Source: three-view drawing plus pictorial views. Frame: mm from the lowest corner of the part. A direction names the side the tool comes from. Round coordinates to 2 decimals unless told otherwise and drop trailing zeros. Write each loop counter-clockwise with the first axis right and the second up, starting at its lowest first coordinate (ties: lowest second). Pieces come first, ordered by that corner, then holes.
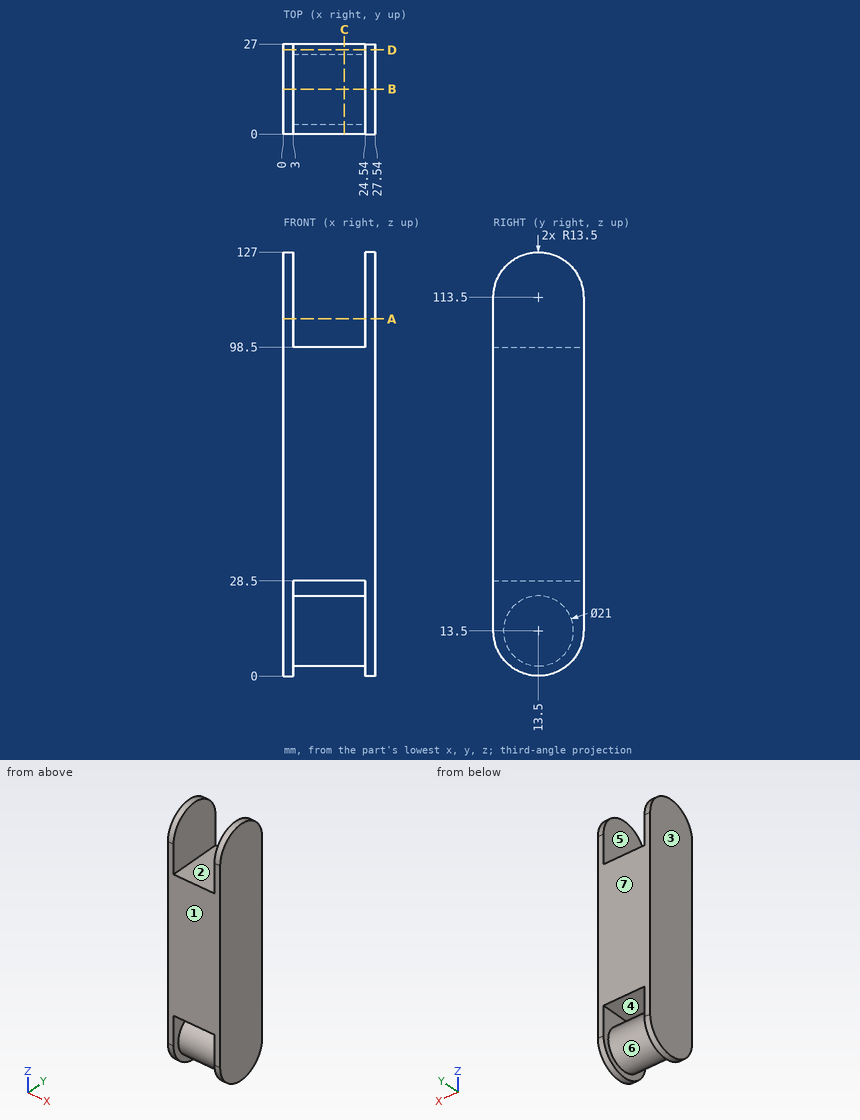
1) Section C-C on x = 18.25. Output: boundary loops of the cut face in (y, z), plus the area to 3 significant figures.
2) Reachability of the marked faces 5, 6 and 7 from +Z, -Z, +X, -X, +Y, -Y: full face, straight path, thin tool, end or side. Return the list, or none.
3) Section D-D on y = 25.25. Output: boundary loops of the cut face in (x, z).
4) First-contact query: P1, Ø1.5, axis at x = 7.5, y = 21, coming from the +Z side; P2, Ø3, axis at x = 9.5, y = 21, coming from the -Z side. Flat tips, straight axial feed; report the tip coordinate or a pass-through.
5) Section B-B on y = 13.5. Output: boundary loops of the cut face in (x, z).
6) Section A-A on z = 107. Output: boundary loops of the cut face in (x, y).
7) Line query: probe 1 along X at (y, z) = (10.25, 103.5); probe 2 along Z at (x, y) = (13.75, 26.25); probe 3 along Z at (x, y) = (19.25, 9.5). Output: solid intervals per line, ascending.
8) Draft query along X for the marked faces 1, 2, 3 and 4. Return one class per face: pulls with the +X half, pulls with the -X half, needs draft (parallel to the pull), parting line crosses it, or undercut.
Filled in:
1. outline: (0, 28.5) - (27, 28.5) - (27, 98.5) - (0, 98.5) - close; circle Ø21 at (13.5, 13.5)
1. area: 2,240 mm2
2. face 5: +Z, +Y, -Y
2. face 6: none
2. face 7: +Z, -Z, +X, -X, +Y
3. outline: (0, 6.85) - (3, 6.85) - (3, 28.5) - (24.54, 28.5) - (24.54, 6.85) - (27.54, 6.85) - (27.54, 120.15) - (24.54, 120.15) - (24.54, 98.5) - (3, 98.5) - (3, 120.15) - (0, 120.15) - close
4. P1: stops at z = 98.5
4. P2: stops at z = 4.88
5. outline: (0, 0) - (3, 0) - (3, 3) - (24.54, 3) - (24.54, 0) - (27.54, 0) - (27.54, 127) - (24.54, 127) - (24.54, 98.5) - (3, 98.5) - (3, 127) - (0, 127) - close; hole (3, 24) - (24.54, 24) - (24.54, 28.5) - (3, 28.5) - close
6. outline: (0, 0) - (3, 0) - (3, 27) - (0, 27) - close; (24.54, 0) - (27.54, 0) - (27.54, 27) - (24.54, 27) - close
7. probe 1: x = 0 to 3, 24.54 to 27.54
7. probe 2: z = 28.5 to 98.5
7. probe 3: z = 3.79 to 23.21, 28.5 to 98.5
8. face 1: needs draft
8. face 2: undercut
8. face 3: pulls with the -X half
8. face 4: undercut
